Build history of the part. All positions in model axes, mm. Face numbers are marked on the shaded views. A direction names the side the tool comes from. Coordinates: 2 decimals unless noted, no trailing zeros. Order: outer loops, then holes, each group sorted by start corner. A loop starts at its lowest first (then second) coordinate and runs counter-clockwise, first axis right, second up. Notation, with made-up numbers: (29.5, 89) - (51.5, 89) arc R14 ccw to (51.5, 111) - close; hole circle Ø2 at (82.25, 83.5). An arc over 180 degrees is marked (long way). Return JSON: item names as keys, results as strings.
from build123d import *

# Parameters (mm, degrees)
SKETCH1_W                       = 25
SKETCH1_H                       = 6.75
BOSS_EXTRUDE1_DEPTH             = 6.5
BOSS_EXTRUDE4_DEPTH             = 6.5
BOSS_EXTRUDE3_REACH             = 6.85
BOSS_EXTRUDE3_DIRECTION_2_REACH = 6.85
SKETCH4_W                       = 2.3
SKETCH4_H                       = 4.5
CUT_EXTRUDE1_DEPTH              = 23
SKETCH6_R                       = 2.55
CUT_EXTRUDE2_DEPTH              = 10
BOSS_EXTRUDE5_DEPTH             = 1.475
CUT_EXTRUDE3_DEPTH              = 3
SKETCH9_R                       = 0.56
CUT_EXTRUDE4_DEPTH              = 9.7
BOSS_EXTRUDE6_DEPTH             = 0.25


with BuildPart() as part:
    # Sketch1 → Boss-Extrude1 (new body)
    with BuildSketch(Plane(origin=(0, 0, 0), x_dir=(1, 0, 0), z_dir=(0, 1, 0))):
        with Locations((12.5, -3.375)):
            Rectangle(SKETCH1_W, SKETCH1_H)
    extrude(amount=BOSS_EXTRUDE1_DEPTH)

    # Sketch5 → Boss-Extrude4 (add)
    with BuildSketch(Plane(origin=(0, 6.5, 0), x_dir=(1, 0, 0), z_dir=(0, 1, 0))):
        Polygon((-5.600297611, -3.375), (-2.800148806, -8.225), (2.800148806, -8.225), (5.600297611, -3.375), (2.800148806, 1.475), (-2.800148806, 1.475), align=None)
    extrude(amount=-BOSS_EXTRUDE4_DEPTH)

    # Boss-Extrude3: up to this face of the body (flat: up to its plane)
    boss_extrude3_end = Plane(part.part.faces().sort_by_distance((0, 3.25, -1.475))[0])
    # Sketch3 → Boss-Extrude3 (add, up to the picked face)
    with BuildSketch(Plane.XY.offset(3.375), mode=Mode.PRIVATE) as boss_extrude3_sk1:
        Polygon((21.275684175, 14.155521181), (26.183820092, 15.109566157), (30, -4.522977512), (25.091864083, -5.477022488), align=None)
    boss_extrude3_tool1 = split(extrude(boss_extrude3_sk1.sketch, amount=-BOSS_EXTRUDE3_REACH, mode=Mode.PRIVATE), bisect_by=boss_extrude3_end, keep=Keep.BOTH, mode=Mode.PRIVATE)
    add(boss_extrude3_tool1.solids().sort_by_distance((25.637842, 4.816272, 3.375))[0])

    # Boss-Extrude3 direction 2: up to this face of the body (flat: up to its plane)
    boss_extrude3_direction_2_end = Plane(part.part.faces().sort_by_distance((0, 3.25, 8.225))[0])
    # Sketch3 → Boss-Extrude3 direction 2 (add, up to the picked face)
    with BuildSketch(Plane.XY.offset(3.375), mode=Mode.PRIVATE) as boss_extrude3_direction_2_sk1:
        Polygon((21.275684175, 14.155521181), (26.183820092, 15.109566157), (30, -4.522977512), (25.091864083, -5.477022488), align=None)
    boss_extrude3_direction_2_tool1 = split(extrude(boss_extrude3_direction_2_sk1.sketch, amount=BOSS_EXTRUDE3_DIRECTION_2_REACH, mode=Mode.PRIVATE), bisect_by=boss_extrude3_direction_2_end, keep=Keep.BOTH, mode=Mode.PRIVATE)
    add(boss_extrude3_direction_2_tool1.solids().sort_by_distance((25.637842, 4.816272, 3.375))[0])

    # Sketch4 → Cut-Extrude1 (cut)
    with BuildSketch(Plane(origin=(-1.876769127, 9.65514015, 0), x_dir=(0.981627183, 0.190808995, 0), z_dir=(-0.190808995, 0.981627183, 0))):
        with Locations((27.435790708, -3.375)):
            Rectangle(SKETCH4_W, SKETCH4_H)
    extrude(amount=-CUT_EXTRUDE1_DEPTH, mode=Mode.SUBTRACT)

    # Sketch6 → Cut-Extrude2 (cut)
    with BuildSketch(Plane(origin=(0, 6.5, 0), x_dir=(1, 0, 0), z_dir=(0, 1, 0))):
        with Locations((0, -3.335615973)):
            Circle(SKETCH6_R)
    extrude(amount=-CUT_EXTRUDE2_DEPTH, mode=Mode.SUBTRACT)

    # Sketch7 → Boss-Extrude5 (add)
    with BuildSketch(Plane(origin=(0, 0, -1.475), x_dir=(-1, 0, 0), z_dir=(0, 0, -1))):
        Polygon((-2.800148806, 0), (-24.027238758, 0), (-25.091864083, -5.477022488), (-30, -4.522977512), (-26.183820092, 15.109566157), (-21.275684175, 14.155521181), (-22.763766749, 6.5), (-2.800148806, 6.5), align=None)
    extrude(amount=-BOSS_EXTRUDE5_DEPTH)

    # Sketch8 → Cut-Extrude3 (cut)
    with BuildSketch(Plane(origin=(0, 0, 0), x_dir=(-1, 0, 0), z_dir=(0, -1, 0))):
        Polygon((-4.67653718, -11.475), (4.67653718, -11.475), (9.353074361, -3.375), (4.67653718, 4.725), (-4.67653718, 4.725), (-9.353074361, -3.375), align=None)
    extrude(amount=-CUT_EXTRUDE3_DEPTH, mode=Mode.SUBTRACT)

    # Sketch9 → Cut-Extrude4 (cut)
    with BuildSketch(Plane(origin=(0, 0, -1.475), x_dir=(-1, 0, 0), z_dir=(0, 0, -1))):
        with Locations((-28.584915246, -3.269967081)):
            Circle(SKETCH9_R)
        with Locations((-27.917083762, 0.165728061)):
            Circle(SKETCH9_R)
    extrude(amount=-CUT_EXTRUDE4_DEPTH, mode=Mode.SUBTRACT)

    # Sketch10 → Boss-Extrude6 (add)
    with BuildSketch(Plane.XY.offset(6.75)):
        Polygon((11.821517388, 5.121255448), (12.792571074, 5.121255448), (12.792571074, 1.621255448), (12.164365946, 1.621255448), (12.164365946, 4.537922115), (11.446417228, 4.537922115), align=None)
        Polygon((14.513825081, 5.121255448), (15.484878766, 5.121255448), (15.484878766, 1.621255448), (14.856673638, 1.621255448), (14.856673638, 4.537922115), (14.13872492, 4.537922115), align=None)
        Polygon((17.234878766, 5.210999038), (17.8182121, 5.210999038), (17.672378766, 4.537922115), (18.215748157, 5.013983814), (18.491289023, 4.537922115), (17.773340305, 4.335999038), (18.491289023, 4.134075961), (18.180692068, 3.647497435), (17.6541496, 4.134075961), (17.8182121, 3.460999038), (17.234878766, 3.460999038), (17.412262581, 4.134075961), (16.873801042, 3.647497435), (16.561801843, 4.134075961), (17.279750561, 4.335999038), (16.561801843, 4.537922115), (16.873801042, 5.036419711), (17.412262581, 4.537922115), align=None)
    extrude(amount=BOSS_EXTRUDE6_DEPTH)


solid = part.part
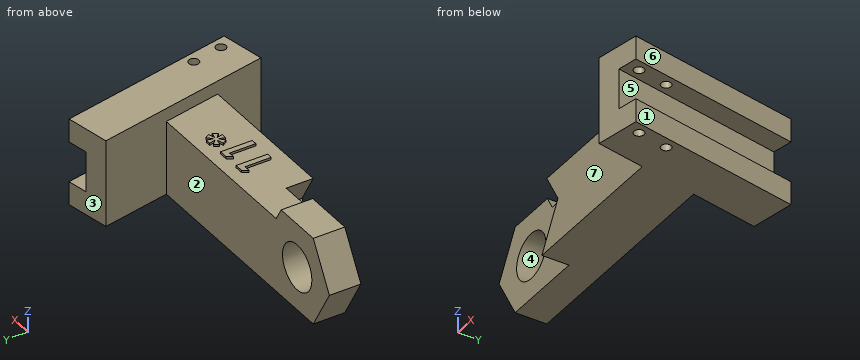
1. Cut at C-C on y = -1.5. Give the cut face in (x, z) (3 decimals).
Check values:
{"outline": "(24.319, -1.475) - (29.412, -1.475) - (29.412, 1.125) - (27.069, 1.125) - (27.069, 5.625) - (29.412, 5.625) - (29.412, 8.225) - (24.319, 8.225) - close"}
2. Tool access for the marked faces 5, 6 and 7: list every direction of +Z, -Z, +X, -X, +Y, -Y with a clear straight run to the whole face (end or side of a thin tool).
Check values:
{"face 5": "+X, +Y", "face 6": "+Z, -Z, +X, +Y", "face 7": "+Z, -Z, -X, -Y"}
3. Mould opens along X. For the marked faces 1, 2, 3 and 4 say: pulls with the +X half, pulls with the -X half, needs draft (parallel to the pull), parting line crosses it, or undercut.
Check values:
{"face 1": "pulls with the +X half", "face 2": "needs draft", "face 3": "pulls with the -X half", "face 4": "undercut"}
4. Cut at B-B on z = 6.25. Give the cut face in (x, y), plus the area to 3 significant figures.
Check values:
{"outline": "(-3.94, 3) - (7.69, 3) - (7.69, 0) - (24.03, 0) - (25.09, -5.48) - (30, -4.52) - (26.18, 15.11) - (21.28, 14.16) - (22.76, 6.5) - (-3.94, 6.5) - close; hole circle Ø1.12 at (27.92, 0.17); hole circle Ø1.12 at (28.58, -3.27)", "area": "241 mm²"}
5. Probe L1, parallel to Z at x = 0, y = 5.25 (3 decimals); L2, parallel to Z at x = 25.5, y = 7.5 (3 decimals); L3, parallel to Y at x = 6, z = 1.75. List the from-to ranges inside material, lowest first.
Check values:
{"L1": "-1.475 to 0.786, 5.886 to 8.225", "L2": "-1.475 to 1.125, 5.625 to 8.225", "L3": "3 to 6.5"}
6. Cut at D-D on y = 2.25. Give the cut face in (x, z) (3 decimals), plus the area to 3 significant figures.
Check values:
{"outline": "(6.553, -1.475) - (28.683, -1.475) - (28.683, 1.125) - (26.34, 1.125) - (26.34, 5.625) - (28.683, 5.625) - (28.683, 8.225) - (23.59, 8.225) - (23.59, 6.75) - (15.485, 6.75) - (15.485, 7) - (14.857, 7) - (14.857, 6.75) - (12.793, 6.75) - (12.793, 7) - (12.164, 7) - (12.164, 6.75) - (7.405, 6.75) - (9.353, 3.375) - close", "area": "166 mm²"}
7. Drop flat-ended pins along their axis: pin 1 (4 mm diameter, centred on x = 12, z = 1, fed in from -Y); pin 2 (1.5 mm diameter, centred on x = 1.5, z = 6.5, fed in from +Y); pin 3 (1 mm diameter, centred on y = 11, z = 0.5, fed in from +X). Give the stop position or say it passes through.
Check values:
{"pin 1": "y = 0", "pin 2": "y = 6.5", "pin 3": "x = 27.08"}
8. Cut at A-A on x = 0. Give the cut face in (y, z) (3 decimals).
Check values:
{"outline": "(3, -1.475) - (6.5, -1.475) - (6.5, 0.786) - (3, 0.786) - close; (3, 5.886) - (6.5, 5.886) - (6.5, 8.225) - (3, 8.225) - close"}
